Read the model definition and answer for the solid it produces. Units are mm, in the model's axes. Face numbers are marked on the shaded views. Give positions to 0.01 mm unless a question says otherwise; leave off trailing zeros. Loops run counter-clockwise (first coordinate to the right, second up) from the corner with the lowest first, then second, coordinate; pieces in that order, holes last.
(1) Determine the mould class of the marked faces 1, 2, 3 and 4 for opening direction Y: pulls with the +Y half, pulls with the -Y half, needs draft (parallel to the pull), parting line crosses it, or undercut.
(2) This flat-tipped pin is pushed along its axis until it touches: P1, Ø3, axis at x = 31.193, y = 89.457, coming from the +Z side. Where does it stop, or does it pass through?
(3) Straight lines are drawn through the part: probe 1 along X at (y, z) = (61, 15.5); probe 2 along X at (y, z) = (62, 5.5); probe 3 along X at (y, z) = (39, 9.25). For each, find the intervals that lie inside material, in ascending order.
(4) Find section C-C, the plane z = 4.5. State how many separate pieces and enclosed holes the cut face has, then the cut area to 3 significant figures.
(5) Find section A-A, the plane y = 79. Write down the section's boundary in (x, z), then the cut area to 3 significant figures.
(6) Find section B-B, the plane x = 24.5. Write down the section's boundary in (y, z), then the cut area to 3 significant figures.
Autodesk Inventor part; units mm, degrees
ref_plane "YZ Plane" through (0, 0, 0) normal (1, 0, 0) x (0, 1, 0)
ref_plane "XZ Plane" through (0, 0, 0) normal (0, 1, 0) x (-1, 0, 0)
ref_plane "XY Plane" through (0, 0, 0) normal (0, 0, 1) x (1, 0, 0)
sketch "Sketch1" plane through (0, 0, 0) normal (0, 0, 1) x (1, 0, 0)
  line L0 (0, 0) -> (120.65, 0)
  line L1 (120.65, 0) -> (120.65, 113.919)
  line L2 (0, 113.919) -> (0, 0)
  circle A0 centre (11.2141, 60.325) radius 1.9431
  circle A1 centre (60.325, 11.2141) radius 1.9431
  circle A2 centre (109.4359, 60.325) radius 1.9431
  circle A3 centre (60.325, 109.4359) radius 1.9431
  circle A4 centre (60.325, 60.325) radius 37.3888
  circle A5 centre (31.193, 89.457) radius 1.6129
  circle A6 centre (31.193, 31.193) radius 1.6129
  circle A7 centre (89.457, 31.193) radius 1.6129
  circle A8 centre (89.457, 89.457) radius 1.6129
  line L3 (60.325, 113.919) -> (120.65, 113.919)
  line L4 (60.325, 113.919) -> (0, 113.919)
  dimension "d10" = 3.8862
  dimension "d13" = 360
  dimension "d18" = 74.7776
  dimension "d20" = 3.2258
  dimension "d23" = 360
  dimension "d32" = 4.4831
extrude "Extrusion3" add sketch "Sketch1" along normal blind 25.4
properties part number "speakerside"
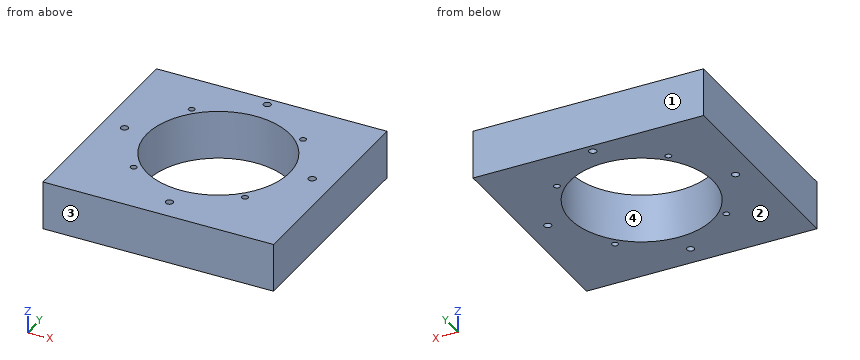
Entries:
1. face 1: pulls with the +Y half
1. face 2: needs draft
1. face 3: pulls with the -Y half
1. face 4: undercut
2. P1: passes through
3. probe 1: x = 0 to 9.39, 13.04 to 22.94, 97.71 to 107.61, 111.26 to 120.65
3. probe 2: x = 0 to 10.23, 12.2 to 22.97, 97.68 to 108.45, 110.42 to 120.65
3. probe 3: x = 0 to 29.61, 91.04 to 120.65
4. separate pieces: 1
4. enclosed holes: 9
4. area: 9,270 mm2
5. outline: (0, 0) - (27.93, 0) - (27.93, 25.4) - (0, 25.4) - close; (92.72, 0) - (120.65, 0) - (120.65, 25.4) - (92.72, 25.4) - close
5. area: 1,420 mm2
6. outline: (0, 0) - (49.62, 0) - (49.62, 25.4) - (0, 25.4) - close; (71.03, 0) - (113.92, 0) - (113.92, 25.4) - (71.03, 25.4) - close
6. area: 2,350 mm2
